Could you check a few things on this model? Use its own coordinates, in mm. A direction names the side the tool comes from. Round coordinates to 2 decimals unless told otherwise and drop trailing zeros. Write each loop counter-clockwise with the first axis right and the second up, starting at its lowest first coordinate (ties: lowest second). Pieces come first, ordered by that corner, then holes. Notation, with made-up numbers: (0.5, 65.25) -> (25.5, 65.25) arc R25 ccw to (25.5, 88.25) -> close; hole circle Ø9 at (-1, -12.5). An arc over 180 degrees is marked (long way). Answer in a Markdown table with one row per item.
from build123d import *

# Parameters (mm, degrees)
SKETCH1_R           = 1.55
BOSS_EXTRUDE1_DEPTH = 5
SKETCH2_W           = 29
SKETCH2_H           = 6
CUT_EXTRUDE1_DEPTH  = 2
CHAMFER1_START      = 3
CHAMFER1_DEPTH      = 2
CHAMFER1_START_2    = -30
CHAMFER1_2_DEPTH    = 6
FILLET1_R           = 3
SKETCH3_R           = 1.55
BOSS_EXTRUDE2_DEPTH = 3
CHAMFER2_SIZE2      = 5.196152423
CHAMFER2_SIZE       = 3


with BuildPart() as part:
    # Sketch1 → Boss-Extrude1 (new body)
    with BuildSketch(Plane(origin=(0, 0, 0), x_dir=(1, 0, 0), z_dir=(0, 1, 0))):
        with BuildLine():
            Line((-3.584795955, -2.802095281), (-17.5, 15))
            Line((-17.5, 15), (-17.5, 27))
            ThreePointArc((-17.5, 27), (-16.621320344, 29.121320344), (-14.5, 30))
            Line((-14.5, 30), (14.5, 30))
            ThreePointArc((14.5, 30), (16.621320344, 29.121320344), (17.5, 27))
            Line((17.5, 27), (17.5, 15))
            Line((17.5, 15), (3.584795955, -2.802095281))
            ThreePointArc((3.584795955, -2.802095281), (0, -4.55), (-3.584795955, -2.802095281))
        make_face()
        with Locations(Location((0, 0, 0), (0, 0, 270))):
            Circle(SKETCH1_R, mode=Mode.SUBTRACT)
        with BuildLine():
            Line((12.5, 22), (-12.5, 22))
            ThreePointArc((-12.5, 22), (-14.5, 24), (-12.5, 26))
            Line((-12.5, 26), (12.5, 26))
            ThreePointArc((12.5, 26), (14.5, 24), (12.5, 22))
        make_face(mode=Mode.SUBTRACT)
    extrude(amount=BOSS_EXTRUDE1_DEPTH)

    # Sketch2 → Cut-Extrude1 (cut)
    with BuildSketch(Plane(origin=(0, 5, 0), x_dir=(1, 0, 0), z_dir=(0, 1, 0))):
        with Locations((0, 27)):
            Rectangle(SKETCH2_W, SKETCH2_H)
    extrude(amount=-CUT_EXTRUDE1_DEPTH, mode=Mode.SUBTRACT)

    # Chamfer1: read off the stored shape, not the designer's step
    # Chamfer1 outline → Chamfer1 (add)
    with BuildSketch(Plane(origin=(0, 0, 0), x_dir=(1, 0, 0), z_dir=(0, 1, 0)).offset(CHAMFER1_START)):
        with BuildLine():
            Line((-12.5, 26), (12.5, 26))
            ThreePointArc((12.5, 26), (13.914213562, 25.414213562), (14.5, 24))
            Line((14.5, 24), (14.5, 30))
            Line((14.5, 30), (-14.5, 30))
            Line((-14.5, 30), (-14.5, 24))
            ThreePointArc((-14.5, 24), (-13.914213562, 25.414213562), (-12.5, 26))
        make_face()
    extrude(amount=CHAMFER1_DEPTH)

    # Chamfer1 2 outline → Chamfer1 2 (cut)
    with BuildSketch(Plane.XY.offset(CHAMFER1_START_2)):
        Polygon((-13.5, 5), (-11.5, 3), (11.5, 3), (13.5, 5), align=None)
    extrude(amount=CHAMFER1_2_DEPTH, mode=Mode.SUBTRACT)

    # Fillet1
    fillet1_edges = [part.edges().sort_by_distance(p)[0] for p in [
        (-17.5, 2.5, -15),
        (17.5, 2.5, -15),
    ]]
    fillet(fillet1_edges, radius=FILLET1_R)

    # Sketch3 → Boss-Extrude2 (add)
    with BuildSketch(Plane(origin=(0, 5, 0), x_dir=(1, 0, 0), z_dir=(0, 1, 0))):
        with BuildLine():
            Line((-17.5, 16.033373903), (17.5, 16.033373903))
            ThreePointArc((17.5, 16.033373903), (17.33644189, 15.056338894), (16.863601728, 14.185838553))
            Line((16.863601728, 14.185838553), (3.584795955, -2.802095281))
            ThreePointArc((3.584795955, -2.802095281), (0, -4.55), (-3.584795955, -2.802095281))
            Line((-3.584795955, -2.802095281), (-16.863601728, 14.185838553))
            ThreePointArc((-16.863601728, 14.185838553), (-17.33644189, 15.056338894), (-17.5, 16.033373903))
        make_face()
        with Locations(Location((0, 0, 0), (0, 0, 270))):
            Circle(SKETCH3_R, mode=Mode.SUBTRACT)
    extrude(amount=BOSS_EXTRUDE2_DEPTH)

    # Chamfer2
    chamfer2_edges = [part.edges().sort_by_distance(p)[0] for p in [
        (0, 8, -16.033373903),
    ]]
    chamfer2_side = [part.faces().sort_by_distance(p)[0] for p in [
        (0, 7.94, -16.033373903),
    ]]
    chamfer(chamfer2_edges, length=CHAMFER2_SIZE - 0.0001, length2=CHAMFER2_SIZE2 - 0.0001, reference=chamfer2_side[0])  # a hair under: the kernel refuses the full size


solid = part.part
1) For faces 4 (the face through (0, 5, -20)), 5 (the face through (0, 2, -22)), 6 (the face through (12.5, 4, -27.9)), 7 (the face through (-16.64, 2.46, -29.1)), 8 (the face through (0, 0, -17)), which set-ups out of +Z, -Z, +X, -X, +Y, -Y let a thin tool reach every point of the face, with its end or its side?
Findings:
| item | result |
|---|---|
| face 4 | -Z, +X, -X, +Y |
| face 5 | +Y, -Y |
| face 6 | -Z, +Y |
| face 7 | -Z, -X, +Y, -Y |
| face 8 | +Z, -Z, +X, -X, -Y |
2) Imagine slicing it at B-B, the plane x = 0. Count the separate pieces of the cut face and the enclosed holes in it, plus the area to 3 significant figures.
Findings:
| item | result |
|---|---|
| separate pieces | 3 |
| enclosed holes | 0 |
| area | 174 mm^2 |
3) Thinking about a two-plate mould opening in Z: for faces 1 (the face through (14.5, 2.5, -24)), 2 (the face through (0.06, 3.94, 4.55)), 3 (the face through (0, 8, -5)), which applies, +Z half, -Z half, draft (parallel to the pull), parting line (faces both ways), or undercut?
Findings:
| item | result |
|---|---|
| face 1 | undercut |
| face 2 | +Z half |
| face 3 | draft |
4) For pin 1 (10 mm diameter, centred on x = -7.5, z = -25.5, fed in from +Y); pin 2 (2 mm diameter, centred on x = -3, y = 1.5, fed in from +Z); pin 3 (1.2 mm diameter, centred on x = 5.5, z = -27.5, fed in from +Y), each with a flat end and sliding along its axis, tell me the tip position at first contact or that it passes through.
Findings:
| item | result |
|---|---|
| pin 1 | stops at y = 5 |
| pin 2 | stops at z = 4.09 |
| pin 3 | stops at y = 3 |
5) Imagine slicing it at C-C, the plane y = 6.75. Please give me the cut outline in (x, z).
Findings:
| item | result |
|---|---|
| outline | (-15.94, -13) -> (15.94, -13) -> (3.58, 2.8) arc R4.55 ccw to (-3.58, 2.8) -> close; hole circle Ø3.1 at (0, 0) |
6) Imagine slicing it at A-A, the plane z = -24. Please give me the cut outline in (x, y), plus the area to 3 significant figures.
Findings:
| item | result |
|---|---|
| outline | (-17.5, 0) -> (-14.5, 0) -> (-14.5, 5) -> (-17.5, 5) -> close; (14.5, 0) -> (17.5, 0) -> (17.5, 5) -> (14.5, 5) -> close |
| area | 30.0 mm^2 |
7) Please list where these lines run through material, in increasing order: line 1 (Y direction, x = -5, z = -28); line 2 (X direction, y = 2.5, z = 0); line 3 (Z direction, x = 1, y = 3.5).
Findings:
| item | result |
|---|---|
| line 1 | y = 0 to 3 |
| line 2 | x = -5.78 to -1.55, 1.55 to 5.78 |
| line 3 | z = -22 to -1.18, 1.18 to 4.44 |
